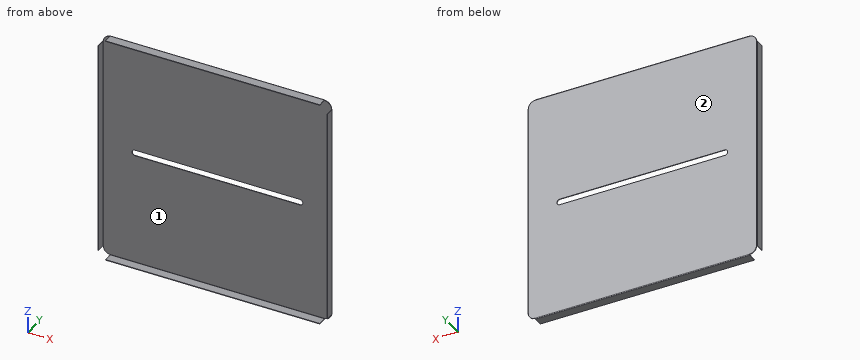
```python
from build123d import *

# Parameters (mm, degrees)
SKETCH1_W                 = 387.38683
SKETCH1_H                 = 391.2598474
BOSS_EXTRUDE1_DEPTH       = 0.035
FILLET1_R                 = 11.811
CONVERT_SOLID1_START      = -0.854
CONVERT_SOLID1_DEPTH      = 0.854
CUT_EXTRUDE1_DEPTH        = 0.889
EDGE_FLANGE1_DEPTH        = 367.6378474
EDGE_FLANGE1_BEND_DEPTH   = 363.76483
EDGE_FLANGE1_BEND_2_DEPTH = 367.6378474
EDGE_FLANGE1_BEND_3_DEPTH = 363.76483


# Read off the part's stored shape, not the designer's step: Convert-Solid1
# Sheet-metal steps are written as plain solids
with BuildPart() as part:
    # Sketch1 → Boss-Extrude1 (new body)
    with BuildSketch(Plane(origin=(0, 0, 0), x_dir=(1, 0, 0), z_dir=(0, 1, 0))):
        Rectangle(SKETCH1_W, SKETCH1_H)
    extrude(amount=BOSS_EXTRUDE1_DEPTH)

    # Fillet1
    fillet1_edges = [part.edges().sort_by_distance(p)[0] for p in [
        (193.693415, 0.0175, -195.6299237),
        (193.693415, 0.0175, 195.6299237),
        (-193.693415, 0.0175, 195.6299237),
        (-193.693415, 0.0175, -195.6299237),
    ]]
    fillet(fillet1_edges, radius=FILLET1_R)

    # Convert-Solid1 outline → Convert-Solid1 (add)
    with BuildSketch(Plane(origin=(0, 0, 0), x_dir=(1, 0, 0), z_dir=(0, 1, 0)).offset(CONVERT_SOLID1_START)):
        with BuildLine():
            ThreePointArc((193.693415, 183.8189237), (190.234053193, 192.170561893), (181.882415, 195.6299237))
            Line((181.882415, 195.6299237), (-181.882415, 195.6299237))
            ThreePointArc((-181.882415, 195.6299237), (-190.234053193, 192.170561893), (-193.693415, 183.8189237))
            Line((-193.693415, 183.8189237), (-193.693415, -183.8189237))
            ThreePointArc((-193.693415, -183.8189237), (-190.234053193, -192.170561893), (-181.882415, -195.6299237))
            Line((-181.882415, -195.6299237), (181.882415, -195.6299237))
            ThreePointArc((181.882415, -195.6299237), (190.234053193, -192.170561893), (193.693415, -183.8189237))
            Line((193.693415, -183.8189237), (193.693415, 183.8189237))
        make_face()
    extrude(amount=CONVERT_SOLID1_DEPTH)

    # Sketch2 → Cut-Extrude1 (cut)
    with BuildSketch(Plane(origin=(0, 0.035, 0), x_dir=(1, 0, 0), z_dir=(0, 1, 0))):
        with BuildLine():
            Line((-140, 5), (140, 5))
            ThreePointArc((140, 5), (145, 0), (140, -5))
            Line((140, -5), (-140, -5))
            ThreePointArc((-140, -5), (-145, 0), (-140, 5))
        make_face()
    extrude(amount=-CUT_EXTRUDE1_DEPTH, mode=Mode.SUBTRACT)

    # Edge-Flange1 section (across the edge) → Edge-Flange1 (add)
    with BuildSketch(Plane(origin=(-194.074415, -0.854, 183.8189237), x_dir=(1, 0, 0), z_dir=(0, 0, -1))):
        with BuildLine():
            Line((-0.889, 0.381), (-0.889, 15))
            Line((-0.889, 15), (0, 15))
            Line((0, 15), (0, 0.381))
            ThreePointArc((0, 0.381), (0.111592316, 0.111592316), (0.381, 0))
            Line((0.381, 0), (0.381, -0.889))
            ThreePointArc((0.381, -0.889), (-0.517025612, -0.517025612), (-0.889, 0.381))
        make_face()
    extrude(amount=EDGE_FLANGE1_DEPTH)

    # Edge-Flange1 section 2 (across the edge) → Edge-Flange1 bend (add)
    with BuildSketch(Plane(origin=(181.882415, -0.854, 196.0109237), x_dir=(0, 0, -1), z_dir=(-1, 0, 0))):
        with BuildLine():
            Line((-0.889, 0.381), (-0.889, 15))
            Line((-0.889, 15), (0, 15))
            Line((0, 15), (0, 0.381))
            ThreePointArc((0, 0.381), (0.111592316, 0.111592316), (0.381, 0))
            Line((0.381, 0), (0.381, -0.889))
            ThreePointArc((0.381, -0.889), (-0.517025612, -0.517025612), (-0.889, 0.381))
        make_face()
    extrude(amount=EDGE_FLANGE1_BEND_DEPTH)

    # Edge-Flange1 section 3 (across the edge) → Edge-Flange1 bend 2 (add)
    with BuildSketch(Plane(origin=(194.074415, -0.854, -183.8189237), x_dir=(-1, 0, 0), z_dir=(0, 0, 1))):
        with BuildLine():
            Line((-0.889, 0.381), (-0.889, 15))
            Line((-0.889, 15), (0, 15))
            Line((0, 15), (0, 0.381))
            ThreePointArc((0, 0.381), (0.111592316, 0.111592316), (0.381, 0))
            Line((0.381, 0), (0.381, -0.889))
            ThreePointArc((0.381, -0.889), (-0.517025612, -0.517025612), (-0.889, 0.381))
        make_face()
    extrude(amount=EDGE_FLANGE1_BEND_2_DEPTH)

    # Edge-Flange1 section 4 (across the edge) → Edge-Flange1 bend 3 (add)
    with BuildSketch(Plane(origin=(-181.882415, -0.854, -196.0109237), x_dir=(0, 0, 1), z_dir=(1, 0, 0))):
        with BuildLine():
            Line((-0.889, 0.381), (-0.889, 15))
            Line((-0.889, 15), (0, 15))
            Line((0, 15), (0, 0.381))
            ThreePointArc((0, 0.381), (0.111592316, 0.111592316), (0.381, 0))
            Line((0.381, 0), (0.381, -0.889))
            ThreePointArc((0.381, -0.889), (-0.517025612, -0.517025612), (-0.889, 0.381))
        make_face()
    extrude(amount=EDGE_FLANGE1_BEND_3_DEPTH)


solid = part.part
```
Geometry: final body of the model. Coordinates: model frame, mm. Face numbers are marked on the shaded views. Round coordinates to 2 decimals unless told otherwise and drop trailing zeros. Loops run counter-clockwise (first coordinate to the right, second up) from the corner with the lowest first, then second, coordinate; pieces in that order, holes last.
Item 1: Section B-B, the plane x = -107. Output: boundary loops of the cut face in (y, z) (3 decimals), plus the area to 3 significant figures.
Checked values:
outline: (-15.854, -196.9) - (-1.235, -196.9) arc R1.27 ccw to (0.035, -195.63) - (0.035, -5) - (-0.854, -5) - (-0.854, -195.63) arc R0.381 cw to (-1.235, -196.011) - (-15.854, -196.011) - close; (-15.854, 196.011) - (-1.235, 196.011) arc R0.381 cw to (-0.854, 195.63) - (-0.854, 5) - (0.035, 5) - (0.035, 195.63) arc R1.27 ccw to (-1.235, 196.9) - (-15.854, 196.9) - close
area: 367 mm2
Item 2: Section D-D, the plane z = -85. Output: boundary loops of the cut face in (x, y) (3 decimals), plus the area to 3 significant figures.
Checked values:
outline: (-194.963, -15.854) - (-194.074, -15.854) - (-194.074, -1.235) arc R0.381 cw to (-193.693, -0.854) - (193.693, -0.854) arc R0.381 cw to (194.074, -1.235) - (194.074, -15.854) - (194.963, -15.854) - (194.963, -1.235) arc R1.27 ccw to (193.693, 0.035) - (-193.693, 0.035) arc R1.27 ccw to (-194.963, -1.235) - close
area: 373 mm2
Item 3: Contact query for flat-ended pins moving along their axis: P1, Ø1, axis at x = -8.5, y = -0.5, coming from the +Z side; P2, Ø1.4, axis at y = -7, z = 196.5, coming from the +X side; P3, Ø1.4, axis at x = -194.5, y = -5, coming from the +Z side. Output: stop coordinate, or through.
Checked values:
P1: stops at z = 196.88
P2: stops at x = 181.88
P3: stops at z = 183.82
Item 4: Mould query, pull axis X, two halves, no side actions, for the marked faces 1 and 2. Classes: released by +X, released by -X, zero draft, split by the parting line, or undercut.
Checked values:
face 1: undercut
face 2: zero draft
Item 5: Section C-C, the plane y = -12. Output: boundary loops of the cut face in (x, z), plus the area to 3 significant figures.
Checked values:
outline: (-194.96, -183.82) - (-194.07, -183.82) - (-194.07, 183.82) - (-194.96, 183.82) - close; (-181.88, -196.9) - (181.88, -196.9) - (181.88, -196.01) - (-181.88, -196.01) - close; (-181.88, 196.01) - (181.88, 196.01) - (181.88, 196.9) - (-181.88, 196.9) - close; (194.07, -183.82) - (194.96, -183.82) - (194.96, 183.82) - (194.07, 183.82) - close
area: 1,300 mm2
Item 6: Section A-A, the plane z = 0. Output: boundary loops of the cut face in (x, y) (3 decimals).
Checked values:
outline: (-194.963, -15.854) - (-194.074, -15.854) - (-194.074, -1.235) arc R0.381 cw to (-193.693, -0.854) - (-145, -0.854) - (-145, 0.035) - (-193.693, 0.035) arc R1.27 ccw to (-194.963, -1.235) - close; (145, -0.854) - (193.693, -0.854) arc R0.381 cw to (194.074, -1.235) - (194.074, -15.854) - (194.963, -15.854) - (194.963, -1.235) arc R1.27 ccw to (193.693, 0.035) - (145, 0.035) - close
Item 7: Line query: L1, parallel to Z at x = 118.5, y = -15; L2, parallel to X at y = -1.5, z = -160.5; L3, parallel to Y at x = 62.5, z = -160.5 (3 decimals). Output: solid intervals per line, ascending.
Checked values:
L1: z = -196.9 to -196.01, 196.01 to 196.9
L2: x = -194.96 to -194.07, 194.07 to 194.96
L3: y = -0.854 to 0.035
